from build123d import *

# Parameters (mm, degrees)
BOSS_EXTRUDE1_DEPTH = 1.5
SKETCH2_W           = 22.2
SKETCH2_H           = 22.2
SKETCH2_W_2         = 20.2
SKETCH2_H_2         = 20.2
BOSS_EXTRUDE2_DEPTH = 1
SKETCH3_W           = 18.2
SKETCH3_H           = 18.2
CUT_EXTRUDE1_DEPTH  = 27.215453458
FILLET1_R           = 2


with BuildPart() as part:
    # Sketch1 → Boss-Extrude1 (new body)
    with BuildSketch(Plane.XY):
        Polygon((-18, -17.5), (-12.5, -17.5), (-12.5, -19), (-6, -19), (-6, -17.5), (6, -17.5), (6, -19), (12.5, -19), (12.5, -17.5), (18, -17.5), (18, 17.5), (12.5, 17.5), (12.5, 19), (6, 19), (6, 17.5), (-6, 17.5), (-6, 19), (-12.5, 19), (-12.5, 17.5), (-18, 17.5), align=None)
    extrude(amount=BOSS_EXTRUDE1_DEPTH)

    # Sketch2 → Boss-Extrude2 (add)
    with BuildSketch(Plane.XY.offset(1.5)):
        Rectangle(SKETCH2_W, SKETCH2_H)
        Rectangle(SKETCH2_W_2, SKETCH2_H_2, mode=Mode.SUBTRACT)
    extrude(amount=BOSS_EXTRUDE2_DEPTH)

    # Sketch3 → Cut-Extrude1 (cut, through all)
    with BuildSketch(Plane.XY.offset(1.5)):
        Rectangle(SKETCH3_W, SKETCH3_H)
    extrude(amount=-CUT_EXTRUDE1_DEPTH, mode=Mode.SUBTRACT)

    # Fillet1
    fillet1_edges = [part.edges().sort_by_distance(p)[0] for p in [
        (18, 17.5, 0.75),
        (18, -17.5, 0.75),
        (-18, -17.5, 0.75),
        (-18, 17.5, 0.75),
    ]]
    fillet(fillet1_edges, radius=FILLET1_R)


solid = part.part
Could you check a few things on this model? Use its own coordinates, in mm. A direction names the side the tool comes from. Round coordinates to 2 decimals unless told otherwise and drop trailing zeros. Write each loop counter-clockwise with the first axis right and the second up, starting at its lowest first coordinate (ties: lowest second). Pieces come first, ordered by that corner, then holes. Notation, with made-up numbers: (59, 62.25) - (103, 62.25) arc R25 cw to (103, 92.25) - close; hole circle Ø8 at (-38.5, 27.5). An arc over 180 degrees is marked (long way). Put each result on its own line as item: value. Start each with the question number.
(1) For faces 1 (the flat face through (0, -10.1, 2)), 2 (the flat face through (11.1, 0, 2)), 3 (the flat face through (-6, -18, 1)), 4 (the flat face through (14, 17.5, 1)), 5 (the flat face through (0, -11.1, 2)), which set-ups out of +Z, -Z, +X, -X, +Y, -Y let a thin tool reach every point of the face, with its end or its side?
(2) Will these pins go through, and if not, where does the flat tip stop? pin 1 (0.8 mm diameter, centred on y = -4, z = 2, fed in from +X); pin 2 (1.5 mm diameter, centred on x = -7.5, y = -1.5, fed in from -Z) (3 decimals); pin 3 (1.2 mm diameter, centred on x = 14.5, z = 1, fed in from +Y); pin 4 (0.8 mm diameter, centred on y = -18, z = 0.5, fed in from -X).
(3) I want a section at C-C, the plane y = 6. Please give me the cut outline in (x, z).
(4) I want a section at B-B, the plane z = 1.95. Please give me the cut outline in (x, y).
(5) I want a section at A-A, the plane x = 8.5. Please give me the cut outline in (y, z), plus the area to 3 significant figures.
(6) I want a section at D-D, the plane y = -14.5. Please give me the cut outline in (x, z), plus the area to 3 significant figures.
(7) Thinking about a two-plate mould opening in X: for faces 6 (the flat face through (-11.1, 0, 2)), 7 (the flat face through (12.5, -18, 1)), 8 (the flat face through (0, 17.5, 1)), which applies, released by +X, released by -X, zero draft, split by the parting line, or undercut?
(8) I need wall thicknesses on probe 1 along X at (y, z) = (0, 1.9); probe 2 along X at (y, z) = (8, 0.7). Which ranges of each line are inside material? Lowest first, please.
Here are the results:
1. face 1: +Z
1. face 2: +Z, +X, +Y, -Y
1. face 3: +Z, -Z, -Y
1. face 4: +Z, -Z, +X, +Y
1. face 5: +Z, +X, -X, -Y
2. pin 1: stops at x = 11.1
2. pin 2: passes through
2. pin 3: stops at y = 17.5
2. pin 4: stops at x = -12.5
3. outline: (-18, 0) - (-9.1, 0) - (-9.1, 1.5) - (-10.1, 1.5) - (-10.1, 2.5) - (-11.1, 2.5) - (-11.1, 1.5) - (-18, 1.5) - close; (9.1, 0) - (18, 0) - (18, 1.5) - (11.1, 1.5) - (11.1, 2.5) - (10.1, 2.5) - (10.1, 1.5) - (9.1, 1.5) - close
4. outline: (-11.1, -11.1) - (11.1, -11.1) - (11.1, 11.1) - (-11.1, 11.1) - close; hole (-10.1, -10.1) - (10.1, -10.1) - (10.1, 10.1) - (-10.1, 10.1) - close
5. outline: (-19, 0) - (-9.1, 0) - (-9.1, 1.5) - (-10.1, 1.5) - (-10.1, 2.5) - (-11.1, 2.5) - (-11.1, 1.5) - (-19, 1.5) - close; (9.1, 0) - (19, 0) - (19, 1.5) - (11.1, 1.5) - (11.1, 2.5) - (10.1, 2.5) - (10.1, 1.5) - (9.1, 1.5) - close
5. area: 31.7 mm^2
6. outline: (-18, 0) - (18, 0) - (18, 1.5) - (-18, 1.5) - close
6. area: 54.0 mm^2
7. face 6: released by -X
7. face 7: released by +X
7. face 8: undercut
8. probe 1: x = -11.1 to -10.1, 10.1 to 11.1
8. probe 2: x = -18 to -9.1, 9.1 to 18
